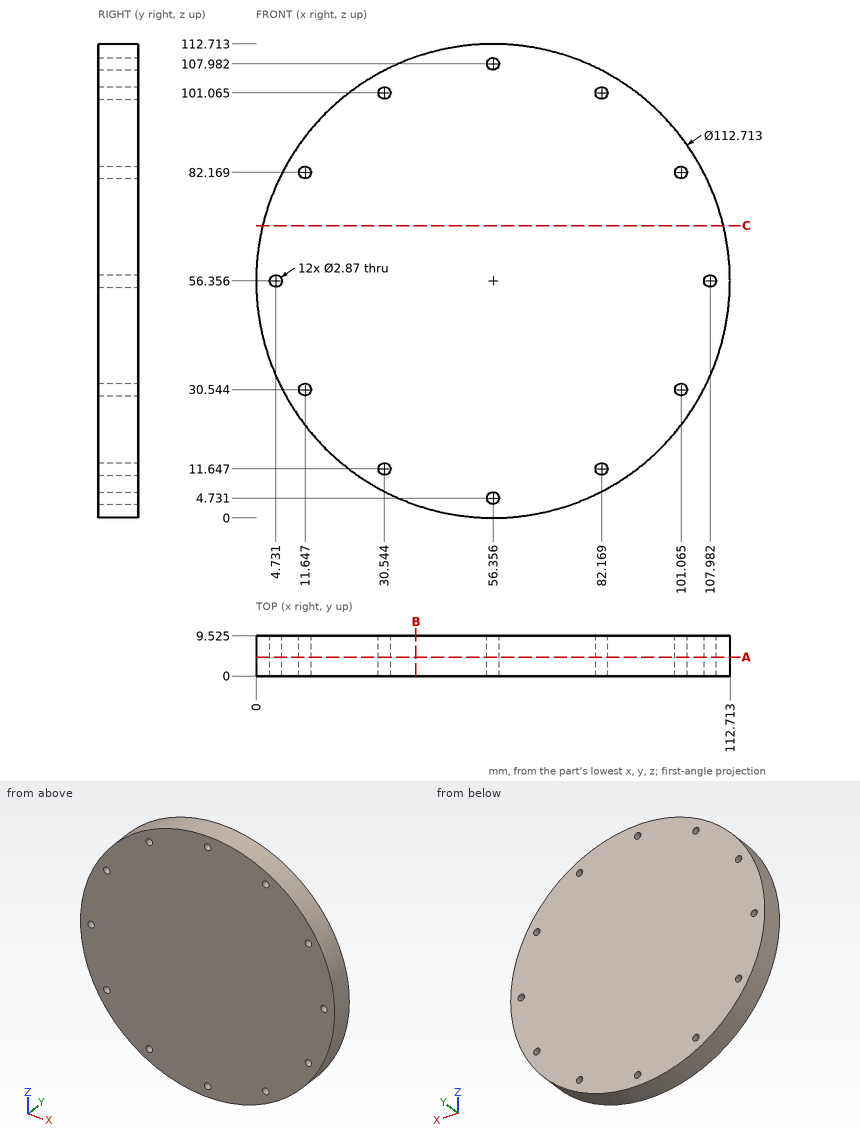
Verification items for this drawing (mm, ordinates from the low corner). Coordinates: 2 decimals unless noted, no trailing zeros. Order: outer loops, then holes, each group sorted by start corner. A loop starts at its lowest first (then second) coordinate and runs counter-clockwise, first axis right, second up.
Q1. Thickness scan on probe 1 along Z at (x, y) = (81.5, 6.75) (1 decimal); probe 2 along X at (y, z) = (0.5, 5.5) (1 decimal); probe 3 along Z at (x, y) = (46.5, 5.5) (1 decimal). Record the ranges inside material, lowest first.
Reply:
probe 1: z = 5.9 to 10.4, 12.9 to 99.8, 102.3 to 106.8
probe 2: x = 32.1 to 55.1, 57.6 to 80.6
probe 3: z = 0.9 to 111.8
Q2. Sectioned sample at A-A on y = 4.5. Give the number of separate pieces and of enclosed holes in the cut face, and give its area (3 significant figures).
Reply:
separate pieces: 1
enclosed holes: 12
area: 9,900 mm2
Q3. Sectioned sample at B-B on x = 38. Record the cut outline in (y, z) (1 decimal), and give its area (4 significant figures).
Reply:
outline: (0, 3.1) - (9.5, 3.1) - (9.5, 109.6) - (0, 109.6) - close
area: 1,015 mm2
Q4. Sectioned sample at C-C on z = 69.5. Record the cut outline in (x, y) (1 decimal).
Reply:
outline: (1.6, 0) - (111.2, 0) - (111.2, 9.5) - (1.6, 9.5) - close
Q5. Depth check by flat-ended pin: pin 1 Ø1.7 at (x, z) = (82.17, 101.07) entering from +Y; pin 2 Ø1.5 at (y, z) = (1.5, 97.5) entering from +X (1 decimal); pin 3 Ø2 at (x, y) = (61.5, 6.5) entering from -Z. Enter the tip coordinate at first touch or a pass-through.
Reply:
pin 1: passes through
pin 2: stops at x = 95.7
pin 3: stops at z = 0.15
